Here's how the part is built. I have some questions about the finished solid (model axes, mm). Coordinates: 2 decimals unless noted, no trailing zeros. Loops run counter-clockwise (first coordinate to the right, second up) from the corner with the lowest first, then second, coordinate; pieces in that order, holes last. Notation, with made-up numbers: M 78.5,-5.5 L 110.5,-5.5 A23 ccw 110.5,13.5 Z; hole C 43,42.5 d10. An arc over 180 degrees is marked long. Use CSV: the item, a comma, the result in double quotes. Start each with the question number.
Q1. If we section it at C-C (x = -98.5): Please give me the cut outline in (y, z), and give its area (3 significant figures).
Q2. If we section it at D-D (y = 4.25): State how many separate pieces and enclosed holes the cut face has, and give its area (3 significant figures).
Q3. If we section it at A-A (z = 4): Please give me the cut outline in (x, y).
Q4. Please list where these lines run through material, in increasing order: probe 1 along X at (y, z) = (1.95, 143); probe 2 along X at (y, z) = (3.3, 192.5); probe 3 along X at (y, z) = (3.25, -222). Write a range as [from, to].
Q5. If we section it at B-B (x = -34): Please give me the cut outline in (y, z), and give its area (3 significant figures).
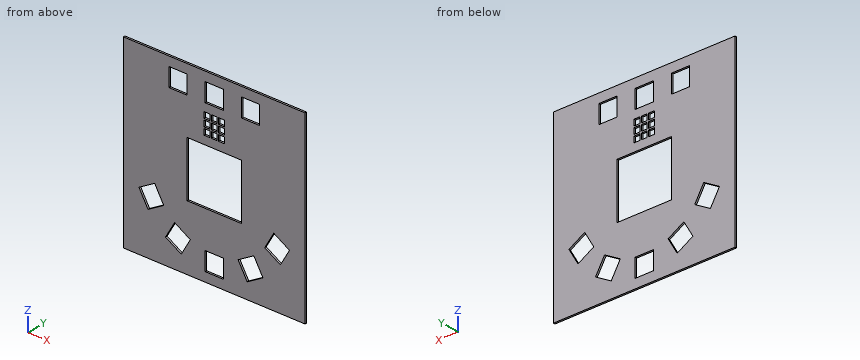
Autodesk Inventor part; units mm, degrees
ref_plane "YZ Plane" through (0, 0, 0) normal (1, 0, 0) x (0, 1, 0)
ref_plane "XZ Plane" through (0, 0, 0) normal (0, 1, 0) x (-1, 0, 0)
ref_plane "XY Plane" through (0, 0, 0) normal (0, 0, 1) x (1, 0, 0)
sketch "Эскиз1" plane through (0, 0, 0) normal (0, 1, 0) x (-1, 0, 0)
  line L0 (28, 97) -> (28, 113)
  line L1 (28, 113) -> (12, 113)
  line L2 (12, 113) -> (12, 97)
  line L3 (12, 97) -> (28, 97)
  line L4 (8, 97) -> (8, 113)
  line L5 (8, 113) -> (-8, 113)
  line L6 (-8, 113) -> (-8, 97)
  line L7 (-8, 97) -> (8, 97)
  line L8 (-12, 97) -> (-12, 113)
  line L9 (-12, 113) -> (-28, 113)
  line L10 (-28, 113) -> (-28, 97)
  line L11 (-28, 97) -> (-12, 97)
  line L12 (-12, 117) -> (-12, 133)
  line L13 (-12, 133) -> (-28, 133)
  line L14 (-28, 133) -> (-28, 117)
  line L15 (-28, 117) -> (-12, 117)
  line L16 (8, 133) -> (-8, 133)
  line L17 (-8, 133) -> (-8, 117)
  line L18 (-8, 117) -> (8, 117)
  line L19 (8, 117) -> (8, 133)
  line L20 (28, 117) -> (28, 133)
  line L21 (28, 133) -> (12, 133)
  line L22 (12, 133) -> (12, 117)
  line L23 (12, 117) -> (28, 117)
  line L24 (28, 137) -> (28, 153)
  line L25 (28, 153) -> (12, 153)
  line L26 (12, 153) -> (12, 137)
  line L27 (12, 137) -> (28, 137)
  line L28 (8, 137) -> (8, 153)
  line L29 (8, 153) -> (-8, 153)
  line L30 (-8, 153) -> (-8, 137)
  line L31 (-8, 137) -> (8, 137)
  line L32 (-12, 137) -> (-12, 153)
  line L33 (-12, 153) -> (-28, 153)
  line L34 (-28, 153) -> (-28, 137)
  line L35 (-28, 137) -> (-12, 137)
  line L36 (-75, 225) -> (-125, 225)
  line L37 (-125, 225) -> (-125, 175)
  line L38 (-125, 175) -> (-75, 175)
  line L39 (-75, 175) -> (-75, 225)
  line L40 (25, 225) -> (-25, 225)
  line L41 (-25, 225) -> (-25, 175)
  line L42 (-25, 175) -> (25, 175)
  line L43 (25, 175) -> (25, 225)
  line L44 (125, 225) -> (75, 225)
  line L45 (75, 225) -> (75, 175)
  line L46 (75, 175) -> (125, 175)
  line L47 (125, 175) -> (125, 225)
  line L48 (75, 75) -> (-75, 75)
  line L49 (-75, 75) -> (-75, -75)
  line L50 (-75, -75) -> (75, -75)
  line L51 (75, -75) -> (75, 75)
  line L52 (-139.0544, -109.1506) -> (-164.0544, -65.8494)
  line L53 (-164.0544, -65.8494) -> (-207.3557, -90.8494)
  line L54 (-207.3557, -90.8494) -> (-182.3557, -134.1506)
  line L55 (-182.3557, -134.1506) -> (-139.0544, -109.1506)
  line L56 (-65.8494, -164.0544) -> (-109.1506, -139.0544)
  line L57 (-109.1506, -139.0544) -> (-134.1506, -182.3557)
  line L58 (-134.1506, -182.3557) -> (-90.8494, -207.3557)
  line L59 (-90.8494, -207.3557) -> (-65.8494, -164.0544)
  line L60 (25, -175) -> (-25, -175)
  line L61 (-25, -175) -> (-25, -225)
  line L62 (-25, -225) -> (25, -225)
  line L63 (25, -225) -> (25, -175)
  line L64 (109.1506, -139.0544) -> (65.8494, -164.0544)
  line L65 (65.8494, -164.0544) -> (90.8494, -207.3557)
  line L66 (90.8494, -207.3557) -> (134.1506, -182.3557)
  line L67 (134.1506, -182.3557) -> (109.1506, -139.0544)
  line L68 (164.0544, -65.8494) -> (139.0544, -109.1506)
  line L69 (139.0544, -109.1506) -> (182.3557, -134.1506)
  line L70 (182.3557, -134.1506) -> (207.3557, -90.8494)
  line L71 (207.3557, -90.8494) -> (164.0544, -65.8494)
  line L72 (-250, -250) -> (-250, 250)
  line L73 (-250, 250) -> (250, 250)
  line L74 (250, 250) -> (250, -250)
  line L75 (250, -250) -> (-250, -250)
  line L76 (-75, 225) -> (-125, 225)
  line L77 (-125, 225) -> (-125, 175)
  line L78 (-125, 175) -> (-75, 175)
  line L79 (-75, 175) -> (-75, 225)
  line L80 (28, 153) -> (12, 153)
  line L81 (12, 153) -> (12, 137)
  line L82 (12, 137) -> (28, 137)
  line L83 (28, 137) -> (28, 153)
  line L84 (28, 133) -> (12, 133)
  line L85 (12, 133) -> (12, 117)
  line L86 (12, 117) -> (28, 117)
  line L87 (28, 117) -> (28, 133)
  line L88 (28, 113) -> (12, 113)
  line L89 (12, 113) -> (12, 97)
  line L90 (12, 97) -> (28, 97)
  line L91 (28, 97) -> (28, 113)
  line L92 (8, 113) -> (-8, 113)
  line L93 (-8, 113) -> (-8, 97)
  line L94 (-8, 97) -> (8, 97)
  line L95 (8, 97) -> (8, 113)
  line L96 (-12, 97) -> (-28, 97)
  line L97 (-28, 97) -> (-28, 113)
  line L98 (-28, 113) -> (-12, 113)
  line L99 (-12, 113) -> (-12, 97)
  line L100 (-12, 117) -> (-28, 117)
  line L101 (-28, 117) -> (-28, 133)
  line L102 (-28, 133) -> (-12, 133)
  line L103 (-12, 133) -> (-12, 117)
  line L104 (-12, 137) -> (-28, 137)
  line L105 (-28, 137) -> (-28, 153)
  line L106 (-28, 153) -> (-12, 153)
  line L107 (-12, 153) -> (-12, 137)
  line L108 (8, 153) -> (-8, 153)
  line L109 (-8, 153) -> (-8, 137)
  line L110 (-8, 137) -> (8, 137)
  line L111 (8, 137) -> (8, 153)
  line L112 (8, 133) -> (-8, 133)
  line L113 (-8, 133) -> (-8, 117)
  line L114 (-8, 117) -> (8, 117)
  line L115 (8, 117) -> (8, 133)
  line L116 (75, 75) -> (-75, 75)
  line L117 (-75, 75) -> (-75, -75)
  line L118 (-75, -75) -> (75, -75)
  line L119 (75, -75) -> (75, 75)
  point P0 (0, 0)
extrude "Выдавливание1" add sketch "Эскиз1" along normal blind 5
properties part number "КВ33.045.001 - Основание" material "Дерево (береза)"
Results below:
1,outline,"M 0,-250 L 5,-250 L 5,-202.94 L 0,-202.94 Z; M 0,-145.2 L 5,-145.2 L 5,175 L 0,175 Z; M 0,225 L 5,225 L 5,250 L 0,250 Z"
1,area,"1,960 mm^2"
2,separate pieces,"1"
2,enclosed holes,"18"
2,area,"205,000 mm^2"
3,outline,"M -250,0 L -75,0 L -75,5 L -250,5 Z; M 75,0 L 250,0 L 250,5 L 75,5 Z"
4,probe 1,"[-250, -28], [-12, -8], [8, 12], [28, 250]"
4,probe 2,"[-250, -125], [-75, -25], [25, 75], [125, 250]"
4,probe 3,"[-250, -25], [25, 250]"
5,outline,"M 0,-250 L 5,-250 L 5,-75 L 0,-75 Z; M 0,75 L 5,75 L 5,250 L 0,250 Z"
5,area,"1,750 mm^2"
